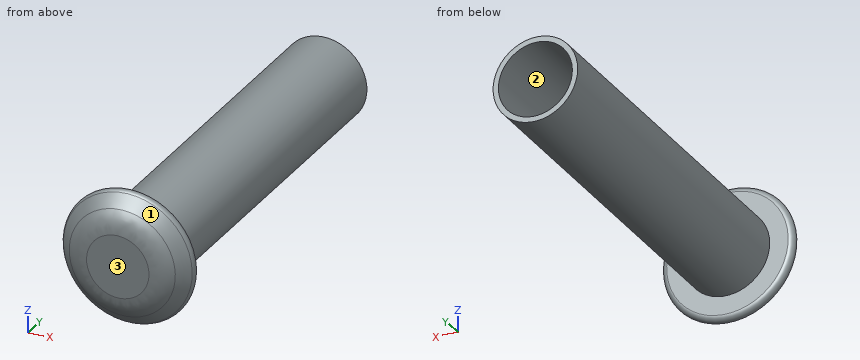
Autodesk Inventor part; units mm, degrees
ref_plane "YZ Plane" through (0, 0, 0) normal (1, 0, 0) x (0, 1, 0)
ref_plane "XZ Plane" through (0, 0, 0) normal (0, 1, 0) x (-1, 0, 0)
ref_plane "XY Plane" through (0, 0, 0) normal (0, 0, 1) x (1, 0, 0)
sketch "Szkic1" plane through (0, 0, 0) normal (0, 1, 0) x (-1, 0, 0)
  circle A0 centre (0, 0) radius 4
  dimension "d0" = 8
extrude "Wyciągnięcie proste1" add sketch "Szkic1" along normal mid plane 35
sketch "Szkic3" plane through (0, 0, 0) normal (1, 0, 0) x (0, 1, 0)
  line L0 (-17.5, 4) -> (-17.5, -4) construction
  line L1 (-17.5, 0) -> (-17.5, 5.7452)
  line L2 (-18.363, 6.0891) -> (-19.3779, 5.0178)
  line L3 (-20.2, 2.9546) -> (-20.2, 0)
  line L4 (-20.2, 0) -> (-17.5, 0)
  arc A0 (-19.3779, 5.0178) -> (-20.2, 2.9546) centre (-17.2, 2.9546) ccw
  arc A1 (-17.5, 5.7452) -> (-18.363, 6.0891) centre (-18, 5.7452) ccw
  line L5 (-17.5, 0) -> (-13.3351, 0) construction
  point P0 (0, 0)
  point P1 (-17.5, 7)
  point P2 (-20.2, 4.15)
  dimension "d3" = 7
  dimension "d4" = 2.7
  dimension "d5" = 4.15
  dimension "d6" = 3
  dimension "d7" = 0.5
revolve "Podstawa" add sketch "Szkic3" angle 360 about axis through (0, -17.5, 0) along (0, 1, 0)
thread "Gwint1"
sketch "Szkic4" plane through (0, 17.5, 0) normal (0, 1, 0) x (1, 0, 0)
  circle A0 centre (0, 0) radius 4
hole "Otwór1" at (0, 17.5, 0) direction (0, -1, 0) diameter 7 depth 15 tip angle 118
properties part number "Rdzeń_wentyla" material "Aluminium AW-7020"
Geometry check sheet. Reference: the model listing, model coordinates, mm. Face numbers are marked on the shaded views. Round coordinates to 2 decimals unless told otherwise and drop trailing zeros. Loops run counter-clockwise (first coordinate to the right, second up) from the corner with the lowest first, then second, coordinate; pieces in that order, holes last. Notation, with made-up numbers: (36, -23.5) - (81, -23.5) arc R35 ccw to (81, 14.5) - close; hole circle Ø11 at (83, -3.5). An arc over 180 degrees is marked (long way). Write each question's results on one line, items separated by ' | '. Start each with the question number.
Q1. Thickness scan on line 1 (Z direction, x = 0, y = 11.5); line 2 (X direction, y = 3, z = -2.5); line 3 (Z direction, x = 0, y = -3.5). Record the ranges inside material, lowest first. Write a range as [from, to].
Q2. Release check for a two-part mould opening along Z. For the marked faces 1, 2 and 3 record: +Z half, -Z half, draft (parallel to the pull), parting line (faces both ways), or undercut.
Q3. Cross-section at B-B on y = 5. Enter the section's corners in (x, z), and give its area (3 significant figures).
Q4. Cross-section at A-A on y = -13. Enter the section's corners in (x, z), and give its area (3 significant figures).
Q5. Gauge pin test, flat ends, axial feed: P1, Ø6, axis at y = -7.5, z = 4.5, coming from the -X side; P2, Ø3, axis at x = 3, y = 12, coming from the +Z side; P3, Ø2, axis at y = 0.5, z = 0.5, coming from the -X side. Record the tip position at first contact, or that the pin passes through.
Answers below:
1) line 1: z = [-4, -3.5], [3.5, 4] | line 2: x = [-3.12, -2.45], [2.45, 3.12] | line 3: z = [-4, 4]
2) face 1: parting line | face 2: undercut | face 3: draft
3) outline: circle Ø8 at (0, 0); hole circle Ø7 at (0, 0) | area: 11.8 mm²
4) outline: circle Ø8 at (0, 0) | area: 50.3 mm²
5) P1: stops at x = -3.71 | P2: stops at z = 3.71 | P3: stops at x = -4
